CAD build for the part. Positions are in the model's coordinates, mm. Face numbers are marked on the shaded views. A direction names the side the tool comes from. Round coordinates to 2 decimals unless told otherwise and drop trailing zeros. Order: outer loops, then holes, each group sorted by start corner. A loop starts at its lowest first (then second) coordinate and runs counter-clockwise, first axis right, second up. Notation, with made-up numbers: (-10, 45.5) - (32, 45.5) arc R23 cw to (32, 68.5) - close; hole circle Ø11 at (24.25, 3.25). An arc over 180 degrees is marked (long way). Use one line per item in the form item = value. Start each with the question number.
from build123d import *

# Parameters (mm, degrees)
F1_DEPTH  = 13.2
F3_DEPTH  = 8
F5_DEPTH  = 88.4390001176
F7_DEPTH  = 48.4308042409
F6_W      = 77
F6_H      = 3
F8_DEPTH  = 12.8
F9_R      = 5
F10_R     = 2
F12_DEPTH = 2
F13_W     = 40.65
F13_H     = 3
F13_W_2   = 12.25
F14_DEPTH = 23.0683441528


# Not quite as in the source:
# - a feature names something its author has since deleted; it is built from what else it names


with BuildPart() as f1:
    # F0 (on Top) → F1 (new body)
    with BuildSketch(Plane.XY):
        with BuildLine():
            Line((-3.2, -10), (4.8, -10))
            Line((4.8, -10), (25, -10))
            Line((25, -10), (25, -33.5))
            ThreePointArc((25, -33.5), (29.9617064043, -36.9938363193), (35.2, -40.0574457714))
            Line((35.2, -40.0574457714), (35.2, -21.1564938874))
            Line((35.2, -21.1564938874), (35.2, -10))
            Line((35.2, -10), (62, -10))
            ThreePointArc((62, -10), (62.8699868465, -17.1376907215), (63.5062507441, -24.3))
            ThreePointArc((63.5062507441, -24.3), (63.7566330876, -28.252847646), (63.9358126513, -32.2095622573))
            ThreePointArc((63.9358126513, -32.2095622573), (64.0273561468, -35.3542873695), (64.0739210442, -38.5))
            ThreePointArc((64.0739210442, -38.5), (64.0571349812, -43.3799777622), (63.9321127792, -48.258382643))
            ThreePointArc((63.9321127792, -48.258382643), (75.0391386854, -48.167385668), (86, -46.3691019944))
            ThreePointArc((86, -46.3691019944), (84.6340109104, -22.9204511896), (79.5, 0))
            Line((79.5, 0), (0, 0))
            Line((0, 0), (-8, 0))
            Line((-8, 0), (-3.2, -10))
        make_face()
        with BuildLine():
            Line((35.2, -21.1564938874), (35.2, -40.0574457714))
            ThreePointArc((35.2, -40.0574457714), (49.1359582734, -45.6647697988), (63.9321127792, -48.258382643))
            ThreePointArc((63.9321127792, -48.258382643), (64.0571349812, -43.3799777622), (64.0739210442, -38.5))
            ThreePointArc((64.0739210442, -38.5), (50.2282447294, -34.8385677857), (37.9, -27.55))
            Line((37.9, -27.55), (37.9, -23.0683441528))
            ThreePointArc((37.9, -23.0683441528), (36.5358784648, -22.1323620803), (35.2, -21.1564938874))
        make_face()
        with BuildLine():
            Line((37.9, -12.8), (37.9, -23.0683441528))
            ThreePointArc((37.9, -23.0683441528), (50.346051903, -29.2676961626), (63.9358126513, -32.2095622573))
            ThreePointArc((63.9358126513, -32.2095622573), (63.7566330876, -28.252847646), (63.5062507441, -24.3))
            ThreePointArc((63.5062507441, -24.3), (51.465613735, -20.0912116842), (41, -12.8))
            Line((41, -12.8), (37.9, -12.8))
        make_face()
        with BuildLine():
            ThreePointArc((63.9358126513, -32.2095622573), (50.346051903, -29.2676961626), (37.9, -23.0683441528))
            Line((37.9, -23.0683441528), (37.9, -27.55))
            ThreePointArc((37.9, -27.55), (50.2282447294, -34.8385677857), (64.0739210442, -38.5))
            ThreePointArc((64.0739210442, -38.5), (64.0273561468, -35.3542873695), (63.9358126513, -32.2095622573))
        make_face()
    extrude(amount=-F1_DEPTH)

    # F2 (on face) → F3 (join)
    with BuildSketch(Plane(origin=(0, 0, -13.2), x_dir=(1, 0, 0), z_dir=(0, 0, -1))):
        Polygon((0.35, 0), (27.35, 0), (27.35, 10), (25, 10), (-3.2, 10), (-8, 0), align=None)
        Polygon((32.85, 10), (32.85, 0), (73.9, 0), (76.2576692783, 10), (62, 10), (35.2, 10), align=None)
        Polygon((32.85, 25.1478344245), (80.4380001176, 25.1478344245), (80.4380001176, 44.1478344245), (44.4380001176, 44.1478344245), (32.85, 38.7561702211), align=None)
    extrude(amount=F3_DEPTH)

    # F4 (on face) → F5 (cut, through all)
    with BuildSketch(Plane.YZ.offset(80.4380001176)):
        with BuildLine():
            Line((0, -18.2), (0, -13.2))
            Line((0, -13.2), (-4.85, -13.2))
            ThreePointArc((-4.85, -13.2), (-7.35, -15.7), (-4.85, -18.2))
            Line((-4.85, -18.2), (0, -18.2))
        make_face()
        with BuildLine():
            Line((-34.85, -18.2), (-30, -18.2))
            Line((-30, -18.2), (-25.1478344245, -18.2))
            Line((-25.1478344245, -18.2), (-25.1478344245, -13.2))
            Line((-25.1478344245, -13.2), (-30, -13.2))
            Line((-30, -13.2), (-34.85, -13.2))
            ThreePointArc((-34.85, -13.2), (-37.35, -15.7), (-34.85, -18.2))
        make_face()
    extrude(amount=-F5_DEPTH, mode=Mode.SUBTRACT)

    # F6 (on face) → F7 (cut, through all)
    with BuildSketch(Plane(origin=(0, 0, 0), x_dir=(-1, 0, 0), z_dir=(0, 1, 0))):
        with BuildLine():
            Line((-32.85, -13.2), (-27.35, -13.2))
            Line((-27.35, -13.2), (-27.35, -12.2))
            ThreePointArc((-27.35, -12.2), (-30.1, -9.45), (-32.85, -12.2))
            Line((-32.85, -12.2), (-32.85, -13.2))
        make_face()
    extrude(amount=-F7_DEPTH, mode=Mode.SUBTRACT)

    # F6 (on face) → F8 (cut, through all)
    with BuildSketch(Plane(origin=(0, 0, 0), x_dir=(-1, 0, 0), z_dir=(0, 1, 0))):
        with Locations((-35.75, -6.5)):
            Rectangle(F6_W, F6_H)
    extrude(amount=-F8_DEPTH, mode=Mode.SUBTRACT)

    # F9
    f9_edges = [f1.edges().sort_by_distance(p)[0] for p in [
        (69.128835, -10, -13.2),
        (26.175, -10, -13.2),
    ]]
    fillet(f9_edges, radius=F9_R)

    # F10
    f10_edges = [f1.edges().sort_by_distance(p)[0] for p in [
        (86, -46.369102, -6.6),
        (79.5, 0, -6.6),
        (25, -33.5, -6.6),
    ]]
    fillet(f10_edges, radius=F10_R)

    # F11 (on face) → F12 (cut)
    with BuildSketch(Plane(origin=(0, 0, -13.2), x_dir=(1, 0, 0), z_dir=(0, 0, -1))):
        with BuildLine():
            Line((73.4852175089, 0), (78.0194737362, 0))
            ThreePointArc((78.0194737362, 0), (79.2135753482, 0.39559315), (79.9352985421, 1.4258786598))
            ThreePointArc((79.9352985421, 1.4258786598), (80.7380621658, 4.2052082165), (81.4852175089, 7))
            Line((81.4852175089, 7), (75.5503684948, 7))
            Line((75.5503684948, 7), (75.0434696, 4.85))
            Line((75.0434696, 4.85), (74.9160721206, 4.85))
            Line((74.9160721206, 4.85), (73.4852175089, 0))
        make_face()
    extrude(amount=-F12_DEPTH, mode=Mode.SUBTRACT)

    # F13 (on face) → F14 (cut, through all)
    with BuildSketch(Plane(origin=(0, 0, 0), x_dir=(-1, 0, 0), z_dir=(0, 1, 0))):
        with Locations((-17.575, -6.5)):
            Rectangle(F13_W, F13_H)
        with Locations((-68.125, -6.5)):
            Rectangle(F13_W_2, F13_H)
    extrude(amount=-F14_DEPTH, mode=Mode.SUBTRACT)


solid = f1.part
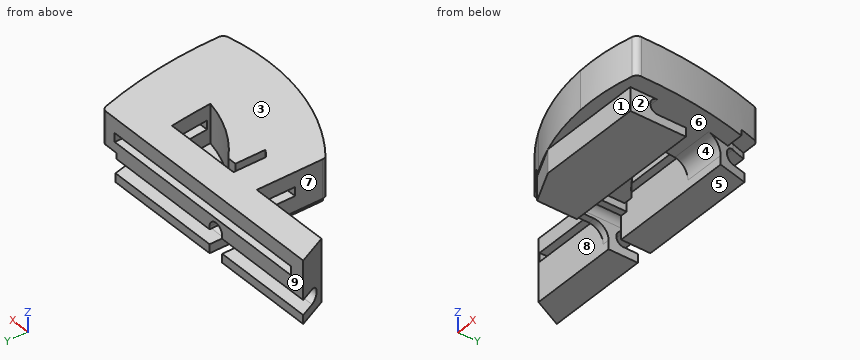
(1) Slice it at A-A (x = 21). Give the cut face in (y, z).
(2) Mould opens along Y. For the marked faces 6, 7, 8 and 9 say: pulls with the +Y half, pulls with the -Y half, needs draft (parallel to the pull), parting line crosses it, or undercut.
(3) Slice it at D-D (x = 60). Give the cut face in (y, z), and give its area (3 significant figures).
(4) Which spindle directions (+Z, -Z, +X, -X, +Y, -Y) get a long thin tool onto all of the face, cutting with end or side? Do the marked faces 1, 2, 3, 4 and 5. Say none if no direction does.
(5) Flat gauge pins, fed straight in: P1, Ø2, axis at y = -23, z = -14.5, coming from the +X side; P2, Ø5.5, axis at y = -23.5, z = -11.5, coming from the -X side; P3, Ø9, axis at y = -30.5, z = -16.5, coming from the +X side; P4, Ø7, axis at y = -10.5, z = -19, coming from the -X side. Where does each tip first touch, or does it go through?
(6) Wall check: line 1 (Z direction, x = 33, y = -3); line 2 (Z direction, x = 68.5, y = -33); line 3 (X direction, y = -38.5, z = -17.75). Give the ranges that are in metal, low to high. Write a range as [from, to].
(7) Slice it at C-C (z = -16.5). Give the cut face in (x, y), and give its area (3 significant figures).
(8) Slice it at B-B (y = -19). Give the cut face in (x, z), and give its area (3 significant figures).
Results list:
q1.outline = (-10, -21.2) - (0, -21.2) - (0, -18.2) - (-4.85, -18.2) arc R2.5 cw to (-4.85, -13.2) - (0, -13.2) - (0, -8) - (-10, -8) - close; (-10, -5) - (0, -5) - (0, 0) - (-10, 0) - close
q2.face_6 = undercut
q2.face_7 = needs draft
q2.face_8 = pulls with the -Y half
q2.face_9 = pulls with the +Y half
q3.outline = (-47.88, -13.2) - (-44.15, -13.2) - (-44.15, -21.2) - (-25.15, -21.2) - (-25.15, -18.2) - (-34.85, -18.2) arc R2.5 cw to (-34.85, -13.2) - (-23.45, -13.2) - (-23.45, 0) - (-47.88, 0) - close; (-10, -21.2) - (0, -21.2) - (0, -18.2) - (-4.85, -18.2) arc R2.5 cw to (-4.85, -13.2) - (0, -13.2) - (0, -8) - (-10, -8) - close; (-10, -5) - (0, -5) - (0, 0) - (-10, 0) - close
q3.area = 564 mm²
q4.face_1 = -Z, +X, -X, -Y
q4.face_2 = -Z, +X, +Y, -Y
q4.face_3 = +Z, +X, -X, +Y, -Y
q4.face_4 = -Z, +X, -X
q4.face_5 = -Z, +X, -X, +Y, -Y
q5.P1 = through
q5.P2 = 25
q5.P3 = 85.73
q5.P4 = -4.64
q6.line_1 = [-21.2, -18.2], [-13.2, -8], [-5, 0]
q6.line_2 = [-21.2, -18.2], [-13.2, 0]
q6.line_3 = [32.85, 80.44]
q7.outline = (-4.54, -7.22) - (-3.2, -10) - (25, -10) - (25, -10.3) - (27.35, -10.3) - (27.35, -7.22) - close; (32.85, -38.76) - (44.44, -44.15) - (80.44, -44.15) - (80.44, -37.22) - (32.85, -37.22) - close; (32.85, -10) - (62, -10) arc R220 cw to (62.04, -10.3) - (76.33, -10.3) - (75.6, -7.22) - (32.85, -7.22) - close
q7.area = 510 mm²
q8.outline = (25, -13.2) - (27.35, -13.2) - (27.35, -12.2) arc R2.75 cw to (32.85, -12.2) - (32.85, -13.2) - (35.2, -13.2) - (35.2, -8) - (25, -8) - close; (25, -5) - (35.2, -5) - (35.2, 0) - (25, 0) - close; (37.9, -13.2) - (49.45, -13.2) - (49.45, 0) - (37.9, 0) - close; (63.06, -13.2) - (84.03, -13.2) - (84.03, 0) - (63.06, 0) - (63.06, -5) - (74.25, -5) - (74.25, -8) - (63.06, -8) - close
q8.area = 482 mm²
